Here's how the part is built. I have some questions about the finished solid (model axes, mm). Face numbers are marked on the shaded views. Coordinates: 2 decimals unless noted, no trailing zeros. Order: outer loops, then holes, each group sorted by start corner. A loop starts at its lowest first (then second) coordinate and runs counter-clockwise, first axis right, second up. Notation, with made-up numbers: M -14,27.25 L 42,27.25 A22 ccw 42,36.25 Z; hole C 54.5,-24 d1. An arc over 180 degrees is marked long. Answer as CSV lines item,"result". Start each with the question number.
```python
from build123d import *

# Parameters (mm, degrees)
SKETCH_1_R          = 44.5
EXTRUDE_1_DEPTH     = 1.5
SKETCH_2_R          = 44.5
SKETCH_2_R_2        = 43
EXTRUDE_2_DEPTH     = 7.5
SKETCH_3_R          = 6
CUT_EXTRUDE_1_DEPTH = 64.572792923


with BuildPart() as part:
    # Эскиз1 → Бобышка-Вытянуть1 (new body)
    with BuildSketch(Plane(origin=(0, 0, 0), x_dir=(1, 0, 0), z_dir=(0, 1, 0))):
        with Locations(Location((0, 0, 0), (0, 0, 270))):
            Circle(SKETCH_1_R)
    extrude(amount=EXTRUDE_1_DEPTH)

    # Эскиз2 → Бобышка-Вытянуть2 (add)
    with BuildSketch(Plane(origin=(0, 1.5, 0), x_dir=(1, 0, 0), z_dir=(0, 1, 0))):
        with Locations(Location((0, 0, 0), (0, 0, 270))):
            Circle(SKETCH_2_R)
        with Locations(Location((0, 0, 0), (0, 0, 270))):
            Circle(SKETCH_2_R_2, mode=Mode.SUBTRACT)
    extrude(amount=EXTRUDE_2_DEPTH)

    # Эскиз3 → Вырез-Вытянуть1 (cut, through all)
    with BuildSketch(Plane.XZ):
        with Locations(Location((0, 0, 0), (0, 0, 270))):
            Circle(SKETCH_3_R)
    extrude(amount=-CUT_EXTRUDE_1_DEPTH, mode=Mode.SUBTRACT)


solid = part.part
```
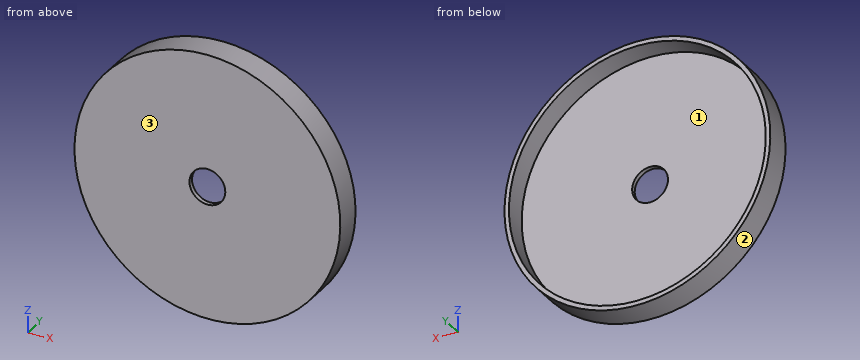
1) I need wall thicknesses on line 1 (X direction, y = 7.75, z = 0); line 2 (X direction, y = 0.9, z = 0); line 3 (Y direction, x = -12, z = 16). Which ranges of each line are inside material? Lowest first, please. Write a range as [from, to].
2) Suppose I cut it at B-B on x = 0. Please give me the cut outline in (y, z), plus the area to 3 significant figures.
3) Will these pins go through, and if not, where does the flat tip stop? pin 1 Ø1 at (x, z) = (-13.5, 10) entering from +Y; pin 2 Ø3 at (y, z) = (1.5, 5.5) entering from -X; pin 3 Ø4 at (x, y) = (7.5, 3) entering from +Z; pin 4 Ø4 at (x, z) = (15, -29) entering from -Y.
4) Suppose I cut it at A-A on z = 0. Please give me the cut outline in (x, y).
5) Suppose I cut it at C-C on y = 6. Please give me the cut outline in (x, z).
6) If we mould it in two halves opening along Z, with no side actions, what happens to the marked faces 1, 2 and 3? For each: released by +Z, released by -Z, zero draft, split by the parting line, or undercut.
7) Suppose I cut it at D-D on x = -21. Please give me the cut outline in (y, z), plus the area to 3 significant figures.
Output:
1,line 1,"[-44.5, -43], [43, 44.5]"
1,line 2,"[-44.5, -6], [6, 44.5]"
1,line 3,"[0, 1.5]"
2,outline,"M 0,-44.5 L 9,-44.5 L 9,-43 L 1.5,-43 L 1.5,-6 L 0,-6 Z; M 0,6 L 1.5,6 L 1.5,43 L 9,43 L 9,44.5 L 0,44.5 Z"
2,area,"138 mm²"
3,pin 1,"y = 1.5"
3,pin 2,"x = -44.32"
3,pin 3,"z = 44.16"
3,pin 4,"y = 0"
4,outline,"M -44.5,0 L -6,0 L -6,1.5 L -43,1.5 L -43,9 L -44.5,9 Z; M 6,0 L 44.5,0 L 44.5,9 L 43,9 L 43,1.5 L 6,1.5 Z"
5,outline,"C 0,0 d89; hole C 0,0 d86"
6,face 1,"undercut"
6,face 2,"split by the parting line"
6,face 3,"zero draft"
7,outline,"M 0,-39.23 L 9,-39.23 L 9,-37.52 L 1.5,-37.52 L 1.5,37.52 L 9,37.52 L 9,39.23 L 0,39.23 Z"
7,area,"143 mm²"
